Design review of the part built by this model. Coordinates are the model's own, in mm. Coordinates: 2 decimals unless noted, no trailing zeros. Write each loop counter-clockwise with the first axis right and the second up, starting at its lowest first coordinate (ties: lowest second). Pieces come first, ordered by that corner, then holes. Notation, with made-up numbers: (-39.75, -39.75) - (-5.75, -39.75) arc R8 cw to (-5.75, -33.75) - close; hole circle Ø1 at (-7, 86.25). An arc over 180 degrees is marked (long way). Answer as a JSON object with one key per item and string values.
```python
from build123d import *

# Parameters (mm, degrees)
SKETCH_1_R = 4


with BuildPart() as part:
    # 扫描1: sweep along a path in 草图2
    with BuildLine(Plane(origin=(0, 0, 0), x_dir=(0, 0, -1), z_dir=(1, 0, 0))) as sweep_1_path:
        Line((0, 0), (5, 0))
        ThreePointArc((5, 0), (12.071067812, -2.928932188), (15, -10))
        Line((15, -10), (15, -11.847012111))
        ThreePointArc((15, -11.847012111), (14.537169507, -14.854070106), (13.191520443, -17.582776475))
        Line((13.191520443, -17.582776475), (-17.177585689, -60.954354864))
        ThreePointArc((-17.177585689, -60.954354864), (-21.659396213, -66.295568657), (-27.000610007, -70.777379181))
        Line((-27.000610007, -70.777379181), (-98.528199032, -120.861536207))
        ThreePointArc((-98.528199032, -120.861536207), (-121.471256486, -128.095454435), (-144.41431394, -120.861536207))
        Line((-144.41431394, -120.861536207), (-291.861681912, -17.617777664))
    # 草图1 → 扫描1 (sweep)
    with BuildSketch(Plane.XY):
        Circle(SKETCH_1_R)
    sweep(path=sweep_1_path.line)


solid = part.part
```
(1) The part is to be moulded in two halves that separate along Y. For faces 1 (the face through (0, 0, 0)), 2 (the face through (-0.06, -17.57, 291.83)), 3 (the face through (-0.867, 3.905, -2.535)), 4 (the face through (-0.521, -65.268, 216.895)), say which applies: pulls with the +Y half, pulls with the -Y half, needs draft (parallel to the pull), parting line crosses it, or undercut.
Solved:
{"face 1": "needs draft", "face 2": "pulls with the +Y half", "face 3": "undercut", "face 4": "parting line crosses it"}
(2) Take a section at A-A, the plane x = 0. Write out the cut boundary in (y, z).
Solved:
{"outline": "(-124.14, 96.23) - (-74.05, 24.71) arc R44 ccw to (-63.25, 13.9) - (-19.88, -16.47) arc R14 ccw to (-11.85, -19) - (-10, -19) arc R14 ccw to (4, -5) - (4, 0) - (-4, 0) - (-4, -5) arc R6 cw to (-10, -11) - (-11.85, -11) arc R6 cw to (-15.29, -9.91) - (-58.66, 20.45) arc R36 cw to (-67.5, 29.29) - (-117.58, 100.82) arc R36 cw to (-117.58, 142.12) - (-14.34, 289.57) - (-20.89, 294.16) - (-124.14, 146.71) arc R44 ccw to start"}
(3) For pin 1 (1.5 mm diameter, centred on x = 1, y = -72.5, fed in from +Z); pin 2 (3 mm diameter, centred on x = 1.5, y = -102, fed in from +Z); pin 3 (1 mm diameter, centred on x = -1, z = 187.5, fed in from +Y), all flat-tipped, find the tip position at first contact; note any pin that passes through.
Solved:
{"pin 1": "stops at z = 221.35", "pin 2": "stops at z = 180.12", "pin 3": "stops at y = -85.59"}
(4) To check wall thickness, follow line 1 (X direction, y = -93.5, z = 60.5); line 2 (Z direction, x = 1, y = -26); line 3 (Z direction, x = -2.75, y = -42.5). State the ranges of each line that lie inside material, in increasing order. Write a range as from..to.
Solved:
{"line 1": "x = -3.95..3.95", "line 2": "z = -12.03..-2.57, 273.14..286.64", "line 3": "z = 0.71..7.8, 251.26..261.39"}
